For this review, take the finished solid that the model builds, in its own axes (mm). A direction names the side the tool comes from. Round coordinates to 2 decimals unless told otherwise and drop trailing zeros. Order: outer loops, then holes, each group sorted by start corner. A loop starts at its lowest first (then second) coordinate and runs counter-clockwise, first axis right, second up. Notation, with made-up numbers: M 59.25,65.25 L 104.25,65.25 A22 cw 104.25,102.25 Z; hole C 49,-9 d4. An arc over 180 degrees is marked long. Put each result on its own line as item: value.
from build123d import *

# Parameters (mm, degrees)
SKETCH_1_R          = 9
EXTRUDE_1_DEPTH     = 1.1
SKETCH_2_R          = 6
EXTRUDE_2_DEPTH     = 6.4
SKETCH_3_R          = 9
EXTRUDE_3_DEPTH     = 1.1
CHAMFER_1_SIZE      = 0.5
SKETCH_4_R          = 2.5
CUT_EXTRUDE_1_DEPTH = 9.6


with BuildPart() as part:
    # 草图1 → 凸台-拉伸1 (new body)
    with BuildSketch(Plane(origin=(0, 0, 0), x_dir=(1, 0, 0), z_dir=(0, 1, 0))):
        Circle(SKETCH_1_R)
    extrude(amount=EXTRUDE_1_DEPTH)

    # 草图2 → 凸台-拉伸2 (add)
    with BuildSketch(Plane(origin=(0, 1.1, 0), x_dir=(1, 0, 0), z_dir=(0, 1, 0))):
        Circle(SKETCH_2_R)
    extrude(amount=EXTRUDE_2_DEPTH)

    # 草图3 → 凸台-拉伸3 (add)
    with BuildSketch(Plane(origin=(0, 7.5, 0), x_dir=(1, 0, 0), z_dir=(0, 1, 0))):
        Circle(SKETCH_3_R)
    extrude(amount=EXTRUDE_3_DEPTH)

    # 倒角1
    chamfer_1_edges = [part.edges().sort_by_distance(p)[0] for p in [
        (-9, 0, 0),
        (-9, 8.6, 0),
    ]]
    chamfer(chamfer_1_edges, length=CHAMFER_1_SIZE)

    # 草图4 → 切除-拉伸1 (cut, through all)
    with BuildSketch(Plane(origin=(0, 8.6, 0), x_dir=(1, 0, 0), z_dir=(0, 1, 0))):
        Circle(SKETCH_4_R)
    extrude(amount=-CUT_EXTRUDE_1_DEPTH, mode=Mode.SUBTRACT)


solid = part.part
(1) Add section C-C on y = 4.75. Give the boundary of the cut face in (x, z).
A:
outline: C 0,0 d12; hole C 0,0 d5
(2) To check wall thickness, follow L1, parallel to Y at x = -6.75, z = -4.25; L2, parallel to Z at x = 0, y = 3. State the ranges of each line that lie inside material, in increasing order.
A:
L1: y = 0 to 1.1, 7.5 to 8.6
L2: z = -6 to -2.5, 2.5 to 6
(3) Insertion check: pin 1 Ø1 at (y, z) = (6.5, 1) entering from -X; pin 2 Ø8 at (x, z) = (5.5, 2.5) entering from -Y; pin 3 Ø1 at (y, z) = (4.5, -4.5) entering from -X; pin 4 Ø1 at (y, z) = (5, -5.5) entering from +X. Each pin has a flat end and moves straight along its axis. Give the tip position at first contact, or say it passes through.
A:
pin 1: stops at x = -5.98
pin 2: stops at y = 0
pin 3: stops at x = -4.47
pin 4: stops at x = 3.32
(4) For faces 1 (the face through (2, 8.6, 2)), 2 (the face through (-6, 4, 0)), list the 3-axis set-ups (+Z, -Z, +X, -X, +Y, -Y) from which the entire face can be reached by the end or side of a thin tool; tool diameter is ignored.
A:
face 1: +Z, -Z, +X, -X, +Y
face 2: none
(5) Draft analysis for pull direction X (two halves, no side actions). For faces 3 (the face through (2, 0, 2)), 4 (the face through (-0.54, 4.36, 2.44)), 5 (the face through (-1.172, 0.796, -8.923)), state which applies: released by +X, released by -X, zero draft, split by the parting line, or undercut.
A:
face 3: zero draft
face 4: undercut
face 5: split by the parting line
(6) Add section B-B on x = 0. Give the boundary of the cut face in (y, z).
A:
outline: M 0,-8.5 L 0.5,-9 L 1.1,-9 L 1.1,-6 L 7.5,-6 L 7.5,-9 L 8.1,-9 L 8.6,-8.5 L 8.6,-2.5 L 0,-2.5 Z; M 0,2.5 L 8.6,2.5 L 8.6,8.5 L 8.1,9 L 7.5,9 L 7.5,6 L 1.1,6 L 1.1,9 L 0.5,9 L 0,8.5 Z
(7) Add section A-A on z = 0. Give the boundary of the cut face in (x, y), then the cut area to 3 significant figures.
A:
outline: M -9,0.5 L -8.5,0 L -2.5,0 L -2.5,8.6 L -8.5,8.6 L -9,8.1 L -9,7.5 L -6,7.5 L -6,1.1 L -9,1.1 Z; M 2.5,0 L 8.5,0 L 9,0.5 L 9,1.1 L 6,1.1 L 6,7.5 L 9,7.5 L 9,8.1 L 8.5,8.6 L 2.5,8.6 Z
area: 72.9 mm2
